from build123d import *

# Parameters (mm, degrees)
EXTRUDE_2_DEPTH          = 11
HOLE_WIZARD_M3_1_D       = 2.5
PATTERN_CIRCULAR_2_COUNT = 3
HOLE_WIZARD_M3_2_D       = 2.5
PATTERN_CIRCULAR_4_COUNT = 3
F_5_0MM_2_D              = 5
PATTERN_CIRCULAR_5_COUNT = 3
CUT_EXTRUDE_1_DEPTH      = 4
FILLET_2_R               = 5
FILLET_4_R               = 5
FILLET_5_R               = 1
FILLET_6_R               = 1


with BuildPart() as part:
    # 스케치1 → 보스-돌출2 (new body)
    with BuildSketch(Plane(origin=(0, 0, 0), x_dir=(1, 0, 0), z_dir=(0, 1, 0))):
        with BuildLine():
            Line((0, -15), (-220.227083718, -9.998002197))
            ThreePointArc((-220.227083718, -9.998002197), (-230.000580731, 0), (-220.227083718, 9.998002197))
            Line((-220.227083718, 9.998002197), (0, 15))
            ThreePointArc((0, 15), (15, 0), (0, -15))
        make_face()
    extrude(amount=EXTRUDE_2_DEPTH)

    # M3 탭을 위한 탭 드릴1 (through all)
    with Locations(Plane(origin=(0, 11, 0), x_dir=(1, 0, 0), z_dir=(0, 1, 0))):
        with Locations((9, 0)):
            hole_wizard_m3_1 = Hole(HOLE_WIZARD_M3_1_D / 2)

    # 원형 패턴2: M3 탭을 위한 탭 드릴1 ×3 about axis
    pattern_circular_2_axis = Axis((0, 0, 0), (0, 1, 0))
    for i in range(1, PATTERN_CIRCULAR_2_COUNT):
        add(hole_wizard_m3_1.rotate(pattern_circular_2_axis, i * 360 / PATTERN_CIRCULAR_2_COUNT), mode=Mode.SUBTRACT)

    # M3 탭을 위한 탭 드릴2 (through all)
    with Locations(Plane(origin=(0, 11, 0), x_dir=(1, 0, 0), z_dir=(0, 1, 0))):
        with Locations((-213.5, 0)):
            hole_wizard_m3_2 = Hole(HOLE_WIZARD_M3_2_D / 2)

    # 원형 패턴4: M3 탭을 위한 탭 드릴2 ×3 about axis
    pattern_circular_4_axis = Axis((-220, 0, 0), (0, 1, 0))
    for i in range(1, PATTERN_CIRCULAR_4_COUNT):
        add(hole_wizard_m3_2.rotate(pattern_circular_4_axis, i * 360 / PATTERN_CIRCULAR_4_COUNT), mode=Mode.SUBTRACT)

    # Ø5.0mm 맞춤핀 구멍2 (through all)
    with Locations(Plane(origin=(0, 11, 0), x_dir=(1, 0, 0), z_dir=(0, 1, 0))):
        with Locations((-9, 0)):
            f_5_0mm_2 = Hole(F_5_0MM_2_D / 2)

    # 원형 패턴5: Ø5.0mm 맞춤핀 구멍2 ×3 about axis
    pattern_circular_5_axis = Axis((0, 0, 0), (0, 1, 0))
    for i in range(1, PATTERN_CIRCULAR_5_COUNT):
        add(f_5_0mm_2.rotate(pattern_circular_5_axis, i * 360 / PATTERN_CIRCULAR_5_COUNT), mode=Mode.SUBTRACT)

    # 스케치26 → 컷-돌출1 (cut)
    with BuildSketch(Plane(origin=(0, 11, 0), x_dir=(1, 0, 0), z_dir=(0, 1, 0))):
        Polygon((-30, 10.317581098), (-205, 6.342821951), (-205, -6.342821951), (-30, -10.317581098), align=None)
    cut_extrude_1 = extrude(amount=-CUT_EXTRUDE_1_DEPTH, mode=Mode.SUBTRACT)

    # 필렛2
    fillet_2_edges = [part.edges().sort_by_distance(p)[0] for p in [
        (-30, 9, -10.317581098),
        (-30, 9, 10.317581098),
        (-205, 9, 6.342821951),
        (-205, 9, -6.342821951),
    ]]
    fillet(fillet_2_edges, radius=FILLET_2_R)

    # 대칭 복사4: 컷-돌출1 across plane
    add(cut_extrude_1.mirror(Plane.ZX.offset(5.5)), mode=Mode.SUBTRACT)

    # 필렛4
    fillet_4_edges = [part.edges().sort_by_distance(p)[0] for p in [
        (-30, 2, 10.317581098),
        (-30, 2, -10.317581098),
        (-205, 2, -6.342821951),
        (-205, 2, 6.342821951),
    ]]
    fillet(fillet_4_edges, radius=FILLET_4_R)

    # 필렛5
    fillet_5_edges = [part.edges().sort_by_distance(p)[0] for p in [
        (-205, 0, 0),
        (-117.613535266, 0, 8.327622808),
        (-117.613535266, 0, -8.327622808),
        (-30, 0, 0),
        (-203.575449365, 0, 4.950259607),
        (-203.575449365, 0, -4.950259607),
        (-31.504837366, 0, 8.778176392),
        (-31.504837366, 0, -8.778176392),
    ]]
    fillet(fillet_5_edges, radius=FILLET_5_R)

    # 필렛6
    fillet_6_edges = [part.edges().sort_by_distance(p)[0] for p in [
        (-117.613535266, 11, 8.327622808),
        (-205, 11, 0),
        (-117.613535266, 11, -8.327622808),
        (-30, 11, 0),
        (-203.575449365, 11, 4.950259607),
        (-203.575449365, 11, -4.950259607),
        (-31.504837366, 11, 8.778176392),
        (-31.504837366, 11, -8.778176392),
    ]]
    fillet(fillet_6_edges, radius=FILLET_6_R)


solid = part.part
The model under review builds one solid part; all positions refer to its coordinate system, in mm. A direction names the side the tool comes from. Give positions to 0.01 mm unless a question says otherwise; leave off trailing zeros. Put each result on its own line as item: value. Start each with the question number.
1. Mouldability with a two-part tool opening along Z and no side actions: class faces 1 (the face through (-79, 0, 13)), 2 (the face through (15, 5, 0)), 3 (the face through (-31.465, 8.479, -8.739)) as released by +Z, released by -Z, zero draft, split by the parting line, or undercut.
2. Clearance check with flat-ended pins moving along their axes: P1, Ø1.5, axis at y = 2, z = 1.5, coming from the -X side; P2, Ø4, axis at x = -64, z = 1, coming from the -Y side; P3, Ø4, axis at y = 9, z = -11.5, coming from the +X side; P4, Ø8, axis at x = 4.5, z = 7.79, coming from the +Y side. State where each tip first meets the part, or that it passes through.
3. For faces 4 (the face through (-31.465, 2.521, -8.739)), 5 (the face through (-203.537, 8.479, 4.989)), 6 (the face through (4.825, 5.423, 5.316)), list the 3-axis set-ups (+Z, -Z, +X, -X, +Y, -Y) from which the entire face can be reached by the end or side of a thin tool; tool diameter is ignored.
4. Wall thickness on probe 1 along X at (y, z) = (2.5, 0.75); probe 2 along X at (y, z) = (6.25, 8); probe 3 along X at (y, z) = (4.5, -6.5): over which ranges is each line inside the solid? List them lowest first.
Determined:
1. face 1: zero draft
1. face 2: split by the parting line
1. face 3: undercut
2. P1: x = -229.97
2. P2: y = 4
2. P3: x = 11.61
2. P4: y = 11
3. face 4: -Y
3. face 5: +Y
3. face 6: +Y, -Y
4. probe 1: -229.97 to -214.5, -212.5 to -205, -30 to -11.38, -6.62 to 8, 10 to 14.98
4. probe 2: -226 to -5.73, -3.27 to 2.01, 6.99 to 12.69
4. probe 3: -227.6 to -224.15, -222.35 to 2.36, 6.64 to 13.52
